from build123d import *

# Parameters (mm, degrees)
ESQUISSE1_R                                      = 38.1
ESQUISSE1_R_2                                    = 11
BOSS_EXTRU_1_DEPTH                               = 15
ESQUISSE2_R                                      = 12.7
ENL_V_MAT_EXTRU_1_DEPTH                          = 7.4
CHAMBRAGE_POUR_VIS_T_TE_RONDE_BOMB_E_D           = 4.3053
CHAMBRAGE_POUR_VIS_T_TE_RONDE_BOMB_E_DEPTH       = 15
CHAMBRAGE_POUR_VIS_T_TE_RONDE_BOMB_E_CBORE_D     = 7.54126
CHAMBRAGE_POUR_VIS_T_TE_RONDE_BOMB_E_CBORE_DEPTH = 2.4638
CHAMBRAGE_POUR_VIS_T_TE_RONDE_BOMB_E_TIP         = 1.293442612
F_1_8_0_124_TROUS_DE_CENTRAGE1_D                 = 3.1496
F_1_8_0_124_TROUS_DE_CENTRAGE1_DEPTH             = 6.35
F_1_8_0_124_TROUS_DE_CENTRAGE1_TIP               = 0.946235303


with BuildPart() as part:
    # Esquisse1 → Boss.-Extru.1 (new body)
    with BuildSketch(Plane.XY):
        with Locations((23.012291104, 8.435887891)):
            Circle(ESQUISSE1_R)
        with Locations((23.012291104, 8.435887891)):
            Circle(ESQUISSE1_R_2, mode=Mode.SUBTRACT)
    extrude(amount=BOSS_EXTRU_1_DEPTH)

    # Esquisse2 → Enlèv. mat.-Extru.1 (cut)
    with BuildSketch(Plane(origin=(0, 0, 0), x_dir=(-1, 0, 0), z_dir=(0, 0, -1))):
        with Locations((-23.012291104, 8.435887891)):
            Circle(ESQUISSE2_R)
    extrude(amount=-ENL_V_MAT_EXTRU_1_DEPTH, mode=Mode.SUBTRACT)

    # Chambrage pour vis à tête ronde bombée #61
    with Locations(Plane.XY.offset(15)):
        with Locations((7.931041104, 34.557379133), (53.174791104, 8.435887891), (7.931041104, -17.68560335)):
            CounterBoreHole(CHAMBRAGE_POUR_VIS_T_TE_RONDE_BOMB_E_D / 2, CHAMBRAGE_POUR_VIS_T_TE_RONDE_BOMB_E_CBORE_D / 2, CHAMBRAGE_POUR_VIS_T_TE_RONDE_BOMB_E_CBORE_DEPTH, depth=CHAMBRAGE_POUR_VIS_T_TE_RONDE_BOMB_E_DEPTH)
            with Locations((0, 0, -(CHAMBRAGE_POUR_VIS_T_TE_RONDE_BOMB_E_DEPTH + CHAMBRAGE_POUR_VIS_T_TE_RONDE_BOMB_E_TIP / 2))):  # 118° drill point
                Cone(0, CHAMBRAGE_POUR_VIS_T_TE_RONDE_BOMB_E_D / 2, CHAMBRAGE_POUR_VIS_T_TE_RONDE_BOMB_E_TIP, mode=Mode.SUBTRACT)

    # 1/8 (0.124) Trous de centrage1
    with Locations(Plane(origin=(0, 0, 0), x_dir=(-1, 0, 0), z_dir=(0, 0, -1))):
        with Locations((-23.012291104, 40.185887891), (-33.871430655, -21.399352819)):
            Hole(F_1_8_0_124_TROUS_DE_CENTRAGE1_D / 2, depth=F_1_8_0_124_TROUS_DE_CENTRAGE1_DEPTH)
            with Locations((0, 0, -(F_1_8_0_124_TROUS_DE_CENTRAGE1_DEPTH + F_1_8_0_124_TROUS_DE_CENTRAGE1_TIP / 2))):  # 118° drill point
                Cone(0, F_1_8_0_124_TROUS_DE_CENTRAGE1_D / 2, F_1_8_0_124_TROUS_DE_CENTRAGE1_TIP, mode=Mode.SUBTRACT)


solid = part.part
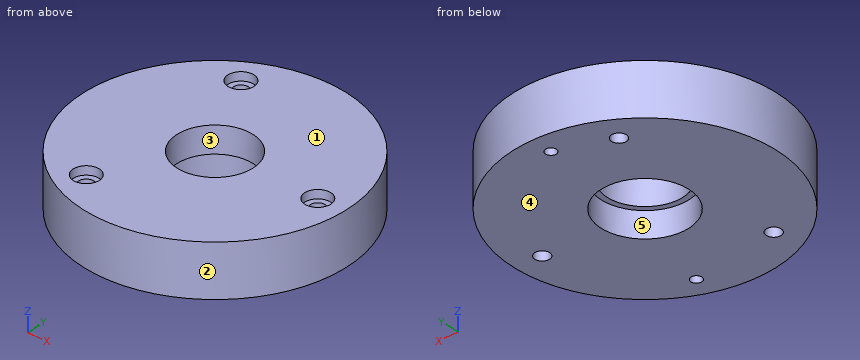
Input: part model. Units: mm. Frame: model coordinates. Face numbers are marked on the shaded views. A direction names the side the tool comes from. Coordinates: 2 decimals unless noted, no trailing zeros. Loops run counter-clockwise (first coordinate to the right, second up) from the corner with the lowest first, then second, coordinate; pieces in that order, holes last.
Q1. Cut plane A-A (y = 1.5). Output: boundary loops of the cut face in (x, z), then the cut area to 3 significant figures.
Q2. Set-up query: the marked faces 4 and 5. Return all of +Z, -Z, +X, -X, +Y, -Y with unobstructed straight access to the full face (end or side cutting, diameter ignored); none if empty.
Q3. Cut plane B-B (z = 13.5). Output: boundary loops of the cut face in (x, y).
Q4. Contact query for flat-ended pins moving along their axis: pin 1 (4 mm diameter, centred on x = 51.5, z = 5, fed in from -Y); pin 2 (1.5 mm diameter, centred on y = 10, z = 11, fed in from -X); pin 3 (7 mm diameter, centred on x = 7.93, y = -17.69, fed in from +Z). Output: stop coordinate, or through.
Q5. Cut plane D-D (y = 15.5). Output: boundary loops of the cut face in (x, z), then the cut area to 3 significant figures.
Q6. Material intervals for line 1 (Y direction, x = 9.5, z = 4.25); line 2 (Y direction, x = 24, z = 2.25); line 3 (Y direction, x = 13, z = 6), sorted ascending.
Q7. Draft query along Y for the marked faces 1, 2 and 3. Return one class per face: +Y half, -Y half, draft (parallel to the pull), parting line (faces both ways), or undercut.
Q8. Cut plane C-C (z = 4.5). Output: boundary loops of the cut face in (x, y).
Working result:
1. outline: (-14.45, 0) - (12.37, 0) - (12.37, 7.4) - (14.47, 7.4) - (14.47, 15) - (-14.45, 15) - close; (31.55, 7.4) - (33.65, 7.4) - (33.65, 0) - (60.48, 0) - (60.48, 15) - (31.55, 15) - close
1. area: 837 mm2
2. face 4: -Z, +X, -X, +Y, -Y
2. face 5: -Z
3. outline: circle Ø76.2 at (23.01, 8.44); hole circle Ø7.54 at (7.93, -17.69); hole circle Ø7.54 at (7.93, 34.56); hole circle Ø22 at (23.01, 8.44); hole circle Ø7.54 at (53.17, 8.44)
4. pin 1: stops at y = -18.95
4. pin 2: stops at x = -15.08
4. pin 3: stops at z = 12.54
5. outline: (-14.43, 0) - (12.46, 0) - (12.46, 7.4) - (14.58, 7.4) - (14.58, 15) - (-14.43, 15) - close; (31.44, 7.4) - (33.57, 7.4) - (33.57, 0) - (60.45, 0) - (60.45, 15) - (31.44, 15) - close
5. area: 839 mm2
6. line 1: y = -27.19 to -19.16, -16.21 to 33.08, 36.03 to 44.06
6. line 2: y = -29.65 to -4.23, 21.1 to 38.96, 41.41 to 46.52
6. line 3: y = -28.33 to 0.62, 16.25 to 45.2
7. face 1: draft
7. face 2: parting line
7. face 3: undercut
8. outline: circle Ø76.2 at (23.01, 8.44); hole circle Ø4.31 at (7.93, -17.69); hole circle Ø4.31 at (7.93, 34.56); hole circle Ø25.4 at (23.01, 8.44); hole circle Ø3.15 at (23.01, 40.19); hole circle Ø3.15 at (33.87, -21.4); hole circle Ø4.31 at (53.17, 8.44)
